```python
from build123d import *

# Parameters (mm, degrees)
F0_R     = 127
F1_DEPTH = 183.69425
F2_T     = -2.54


# Not quite as in the source:
# - a fillet or chamfer that OpenCascade refuses, or shapes differently, is made with other operations: its cross-section is extruded or revolved along the edge and cut away or added


with BuildPart() as f1:
    # F0 (on Front) → F1 (new body)
    with BuildSketch(Plane.XZ):
        Circle(F0_R)
    extrude(amount=F1_DEPTH)

    # F2
    f2_openings = [f1.faces().sort_by_distance(p)[0] for p in [
        (0, -183.69425, 0),
    ]]
    offset(amount=F2_T, openings=f2_openings)

    # F3: fillet of radius 25.4 on 3 edges, made by hand

    # F3_s1 → F3_t2 (revolve)
    with BuildSketch(Plane.XY):
        with BuildLine():
            ThreePointArc((124.46, -27.94), (117.0205122421, -9.9794877579), (99.06, -2.54))
            Line((99.06, -2.54), (124.46, -2.54))
            Line((124.46, -2.54), (124.46, -27.94))
        make_face()
    revolve(axis=Axis((0, -2.54, 0), (0, 1, 0)))

    # F3_s3 → F3_t4 (revolve, cut)
    with BuildSketch(Plane.XY):
        with BuildLine():
            ThreePointArc((127, -25.4), (119.5605122421, -7.4394877579), (101.6, 0))
            Line((101.6, 0), (127, 0))
            Line((127, 0), (127, -25.4))
        make_face()
    revolve(axis=Axis((0, 0, 0), (0, -1, 0)), mode=Mode.SUBTRACT)

    # F3_s5 → F3_t6 (revolve, cut)
    with BuildSketch(Plane.XY):
        with BuildLine():
            ThreePointArc((127, -183.69425), (125.1031423642, -178.3022593463), (124.46, -172.6226466834))
            Line((124.46, -172.6226466834), (124.46, -183.69425))
            Line((124.46, -183.69425), (127, -183.69425))
        make_face()
    revolve(axis=Axis((0, -183.69425, 0), (0, -1, 0)), mode=Mode.SUBTRACT)


solid = f1.part
```
CAD build for the part. Positions are in the model's coordinates, mm. Round coordinates to 2 decimals unless told otherwise and drop trailing zeros. Order: outer loops, then holes, each group sorted by start corner. A loop starts at its lowest first (then second) coordinate and runs counter-clockwise, first axis right, second up. Notation, with made-up numbers: (15, 66.5) - (73, 66.5) arc R18 cw to (73, 100.5) - close; hole circle Ø9 at (56.25, 35). An arc over 180 degrees is marked (long way). Answer as CSV lines item,"result". Start each with the question number.
1. Pull direction X, two halves, no side cores. Call faces 1 (the face through (-1, 0, 1)), 2 (the face through (-27.53, -103.44, -123.98)), 3 (the face through (-1, -2.54, 1)), 4 (the face through (-26.98, -99.27, -121.5)): +X half, -X half, draft (parallel to the pull), parting line (faces both ways), or undercut.
2. Saw through at D-D, the plane y = -14. Write the cut outline in (x, z).
3. Saw through at C-C, the plane y = -122.5. Write the cut outline in (x, z), and give its area (3 significant figures).
4. Saw through at A-A, the plane x = 0. Write the cut outline in (y, z), and give its area (3 significant figures).
5. Saw through at B-B, the plane z = 0. Write the cut outline in (x, y).
6. Drill centre lines: L1, parallel to Z at x = 0, y = -61; L2, parallel to Y at x = 56, z = 10. Where is each one in solid material? Low to high. Write a range as [from, to].
7. Pin check, flat tips, straight feed: pin 1 (12 mm diameter, centred on x = 11.5, y = -38, fed in from +Z); pin 2 (6 mm diameter, centred on x = 65.5, z = -87.5, fed in from +Y); pin 3 (4 mm diameter, centred on x = -85, y = -48, fed in from -Z). Stop position of each tip, or through.
Model answer:
1,face 1,"draft"
1,face 2,"parting line"
1,face 3,"undercut"
1,face 4,"undercut"
2,outline,"circle Ø248.6 at (0, 0); hole circle Ø240.59 at (0, 0)"
3,outline,"circle Ø254 at (0, 0); hole circle Ø248.92 at (0, 0)"
3,area,"2,010 mm²"
4,outline,"(-183.69, -127) - (-25.4, -127) arc R25.4 ccw to (0, -101.6) - (0, 101.6) arc R25.4 ccw to (-25.4, 127) - (-183.69, 127) arc R25.4 ccw to (-172.62, 124.46) - (-27.94, 124.46) arc R25.4 cw to (-2.54, 99.06) - (-2.54, -99.06) arc R25.4 cw to (-27.94, -124.46) - (-172.62, -124.46) arc R25.4 ccw to start"
4,area,"1,550 mm²"
5,outline,"(-127, -183.69) arc R25.4 ccw to (-124.46, -172.62) - (-124.46, -27.94) arc R25.4 cw to (-99.06, -2.54) - (99.06, -2.54) arc R25.4 cw to (124.46, -27.94) - (124.46, -172.62) arc R25.4 ccw to (127, -183.69) - (127, -25.4) arc R25.4 ccw to (101.6, 0) - (-101.6, 0) arc R25.4 ccw to (-127, -25.4) - close"
6,L1,"z = [-127, -124.46], [124.46, 127]"
6,L2,"y = [-2.54, 0]"
7,pin 1,"stops at z = 126.88"
7,pin 2,"stops at y = -0.44"
7,pin 3,"stops at z = -96.12"
